Can you work these out from the model? Positions are in its coordinate system, mm. Face numbers are marked on the shaded views. A direction names the side the tool comes from. Round coordinates to 2 decimals unless told otherwise and drop trailing zeros. Loops run counter-clockwise (first coordinate to the right, second up) from the corner with the lowest first, then second, coordinate; pieces in that order, holes last. Notation, with made-up numbers: (-3.75, 81.5) -> (46.25, 81.5) arc R9 ccw to (46.25, 97.5) -> close; hole circle Ø5 at (47, 28). An arc over 180 degrees is marked (long way). Answer as a JSON object with one key per item and string values.
Autodesk Inventor part; units mm, degrees
ref_plane "YZ Plane" through (0, 0, 0) normal (1, 0, 0) x (0, 1, 0)
ref_plane "XZ Plane" through (0, 0, 0) normal (0, 1, 0) x (-1, 0, 0)
ref_plane "XY Plane" through (0, 0, 0) normal (0, 0, 1) x (1, 0, 0)
sketch "Sketch1" plane through (0, 0, 0) normal (1, 0, 0) x (0, 1, 0)
  line L0 (-26.75, 9.25) -> (26.75, 9.25)
  line L1 (26.75, 9.25) -> (26.75, -9.25)
  line L2 (26.75, -9.25) -> (-26.75, -9.25)
  line L3 (-26.75, -9.25) -> (-26.75, 9.25)
  line L4 (-26.75, 9.25) -> (26.75, -9.25) construction
  line L5 (26.75, 9.25) -> (-26.75, -9.25) construction
  circle A0 centre (15, 0) radius 2.1
  circle A1 centre (-15, 0) radius 2.1
  point P0 (0, 0)
  dimension "d0" = 53.5
  dimension "d1" = 18.5
  dimension "d2" = 4.2
  dimension "d3" = 4.2
  dimension "d4" = 30
  dimension "d5" = 11.75
  dimension "d6" = 9.25
  dimension "d7" = 9.25
extrude "Extrusion1" add sketch "Sketch1" along normal blind 6
sketch "Sketch2" plane through (0, 0, 0) normal (-1, 0, 0) x (0, 0, 1)
  line L0 (-9.25, 26.75) -> (9.25, 26.75)
  line L1 (-9.25, 26.75) -> (9.25, 26.75)
  line L2 (9.25, 26.75) -> (9.25, 20.75)
  line L3 (9.25, 20.75) -> (-9.25, 20.75)
  line L4 (-9.25, 20.75) -> (-9.25, 26.75)
  line L5 (9.25, 26.75) -> (9.25, -26.75)
  line L6 (9.25, -26.75) -> (-9.25, -26.75)
  line L7 (-9.25, -26.75) -> (-9.25, -20.75)
  line L8 (-9.25, -20.75) -> (9.25, -20.75)
  line L9 (9.25, -20.75) -> (9.25, -26.75)
  point P0 (0, 0)
  dimension "d10" = 18.5
  dimension "d11" = 6
  dimension "d12" = 18.5
  dimension "d13" = 6
extrude "Extrusion2" add sketch "Sketch2" along normal blind 20
sketch "Sketch3" plane through (6, 26.75, 9.25) normal (0, 1, 0) x (1, 0, 0)
  circle A0 centre (-20, 9.25) radius 2.1
  line L0 (0, 0) -> (-26, 0)
  line L1 (0, 18.5) -> (0, 0)
  point P0 (-6, 9.25)
  dimension "d16" = 4.2
  dimension "d18" = 20
  dimension "d21" = 9.25
extrude "Extrusion3" cut sketch "Sketch3" against normal blind 100
equation "\"d7\" = d6"
properties part number "End Bracing" material "Aluminum 6061"
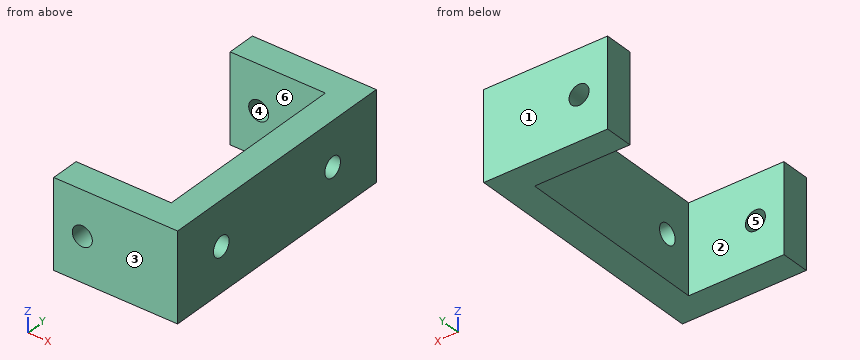
Q1. If I drill on L1, parallel to Y at x = -1, z = -5.5; L2, parallel to Z at x = 3.3, y = -15; L3, parallel to X at y = 22.85, z = 0, over which ranges is the centre line in solid material (lowest first)? Write a range as [from, to].
Determined:
{"L1": "[-26.75, -20.75], [20.75, 26.75]", "L2": "[-9.25, -2.1], [2.1, 9.25]", "L3": "[-20, -16.1], [-11.9, 6]"}
Q2. I want a section at A-A, the plane x = -6.75. Write out the boundary of the cut face in (y, z), then the cut area to 3 significant figures.
Determined:
{"outline": "(-26.75, -9.25) -> (-20.75, -9.25) -> (-20.75, 9.25) -> (-26.75, 9.25) -> close; (20.75, -9.25) -> (26.75, -9.25) -> (26.75, 9.25) -> (20.75, 9.25) -> close", "area": "222 mm²"}
Q3. I want a section at B-B, the plane z = 0. Write out the boundary of the cut face in (x, y), then the cut area to 3 significant figures.
Determined:
{"outline": "(-20, -26.75) -> (-16.1, -26.75) -> (-16.1, -20.75) -> (-20, -20.75) -> close; (-20, 20.75) -> (-16.1, 20.75) -> (-16.1, 26.75) -> (-20, 26.75) -> close; (-11.9, -26.75) -> (6, -26.75) -> (6, -17.1) -> (0, -17.1) -> (0, -20.75) -> (-11.9, -20.75) -> close; (-11.9, 20.75) -> (0, 20.75) -> (0, 17.1) -> (6, 17.1) -> (6, 26.75) -> (-11.9, 26.75) -> close; (0, -12.9) -> (6, -12.9) -> (6, 12.9) -> (0, 12.9) -> close", "area": "460 mm²"}
Q4. I want a section at C-C, the plane y = -15. Write out the boundary of the cut face in (x, z).
Determined:
{"outline": "(0, -9.25) -> (6, -9.25) -> (6, -2.1) -> (0, -2.1) -> close; (0, 2.1) -> (6, 2.1) -> (6, 9.25) -> (0, 9.25) -> close"}
Q5. I want a section at D-D, the plane x = -14. Write out the boundary of the cut face in (y, z), then the cut area to 3 significant figures.
Determined:
{"outline": "(-26.75, -9.25) -> (-20.75, -9.25) -> (-20.75, -2.1) -> (-26.75, -2.1) -> close; (-26.75, 2.1) -> (-20.75, 2.1) -> (-20.75, 9.25) -> (-26.75, 9.25) -> close; (20.75, -9.25) -> (26.75, -9.25) -> (26.75, -2.1) -> (20.75, -2.1) -> close; (20.75, 2.1) -> (26.75, 2.1) -> (26.75, 9.25) -> (20.75, 9.25) -> close", "area": "172 mm²"}
Q6. I'm going to push flat-ended pins straight in: pin 1 (6 mm diameter, centred on x = -14, z = -2, fed in from -Y); pin 2 (5.5 mm diameter, centred on y = 15, z = 0, fed in from -X). Where does each tip first touch, or does it pass through?
Determined:
{"pin 1": "y = -26.75", "pin 2": "x = 0"}
Q7. On a 3-axis mill with a long thin cutter (end or side, diameter ignored), from which of +Z, -Z, +X, -X, +Y, -Y can I reach the whole of each face in a straight line? I mean the marked faces 5 and 6. Say none if no direction works.
Determined:
{"face 5": "+Y, -Y", "face 6": "+Z, -Z, -X"}
Q8. We'd pull the mould along Y, two halves only. Please class the marked faces 1, 2, 3 and 4: pulls with the +Y half, pulls with the -Y half, needs draft (parallel to the pull), parting line crosses it, or undercut.
Determined:
{"face 1": "pulls with the +Y half", "face 2": "undercut", "face 3": "pulls with the -Y half", "face 4": "needs draft"}
